Solid Edge part; units mm, degrees
sketch "Sketch1" plane through (0, 0, 0) normal (0, 0, 1) x (1, 0, 0)
  line L0 (0, 7.35) -> (6.3653, 3.675)
  line L1 (6.3653, 3.675) -> (6.3653, -3.675)
  line L2 (6.3653, -3.675) -> (0, -7.35)
  line L3 (0, -7.35) -> (-6.3653, -3.675)
  line L4 (-6.3653, -3.675) -> (-6.3653, 3.675)
  line L5 (-6.3653, 3.675) -> (0, 7.35)
extrude "Protrusion1" add sketch "Sketch1" along normal blind 6.3
sketch "Sketch2" plane through (0, 0, 6.3) normal (0, 0, 1) x (0.866, 0.5, 0)
  circle A0 centre (0, 0) radius 4
extrude "Cutout1" cut sketch "Sketch2" against normal through all
properties material "Stainless steel"
Could you check a few things on this model? Use its own coordinates, in mm. Round coordinates to 2 decimals unless told otherwise and drop trailing zeros. Write each loop counter-clockwise with the first axis right and the second up, starting at its lowest first coordinate (ties: lowest second). Pieces come first, ordered by that corner, then holes. Notation, with made-up numbers: (10, 29.5) - (62, 29.5) arc R17 cw to (62, 37.5) - close; hole circle Ø6 at (73, -5). An arc over 180 degrees is marked (long way). Use a Markdown table: item, result.
Q1. Thinking about a two-plate mould opening in Y: for faces 1 (the flat face through (-6.365, 0, 3)), 2 (the flat face through (3.227, -5.487, 3.106)), 3 (the cylindrical face through (3.966, 0.521, 3.194)), which applies, released by +Y, released by -Y, zero draft, split by the parting line, or undercut?
Output values:
| item | result |
|---|---|
| face 1 | zero draft |
| face 2 | released by -Y |
| face 3 | undercut |
Q2. I want a section at C-C (z = 3). List the corners of the cut face in (x, y) for me (3 decimals), plus the area to 3 significant figures.
Output values:
| item | result |
|---|---|
| outline | (-6.365, -3.675) - (0, -7.35) - (6.365, -3.675) - (6.365, 3.675) - (0, 7.35) - (-6.365, 3.675) - close; hole circle Ø8 at (0, 0) |
| area | 90.1 mm2 |
Q3. I want a section at B-B (x = 3.25). List the corners of the cut face in (y, z) for me.
Output values:
| item | result |
|---|---|
| outline | (-5.47, 0) - (-2.33, 0) - (-2.33, 6.3) - (-5.47, 6.3) - close; (2.33, 0) - (5.47, 0) - (5.47, 6.3) - (2.33, 6.3) - close |
Q4. Please list where these lines run through material, in increasing order: L1, parallel to X at y = 0, z = 2; L2, parallel to X at y = -3.5, z = 2; L3, parallel to Y at x = 2, z = 1.5.
Output values:
| item | result |
|---|---|
| L1 | -6.37 to -4, 4 to 6.37 |
| L2 | -6.37 to -1.94, 1.94 to 6.37 |
| L3 | -6.2 to -3.46, 3.46 to 6.2 |
Q5. For pin 1 (1.5 mm diameter, centred on x = 4, z = 3, fed in from -Y), with a flat end and sliding along its axis, tell me the tip position at first contact or that it passes through.
Output values:
| item | result |
|---|---|
| pin 1 | y = -5.47 |
Q6. I want a section at A-A (y = 0). List the corners of the cut face in (x, z) for me.
Output values:
| item | result |
|---|---|
| outline | (-6.37, 0) - (-4, 0) - (-4, 6.3) - (-6.37, 6.3) - close; (4, 0) - (6.37, 0) - (6.37, 6.3) - (4, 6.3) - close |
